Could you check a few things on this drawing? It's one solid part, dimensions in mm from its lowest x, y, z. A direction names the side the tool comes from. Coordinates: 2 decimals unless noted, no trailing zeros. Order: outer loops, then holes, each group sorted by start corner. A loop starts at its lowest first (then second) coordinate and runs counter-clockwise, first axis right, second up.
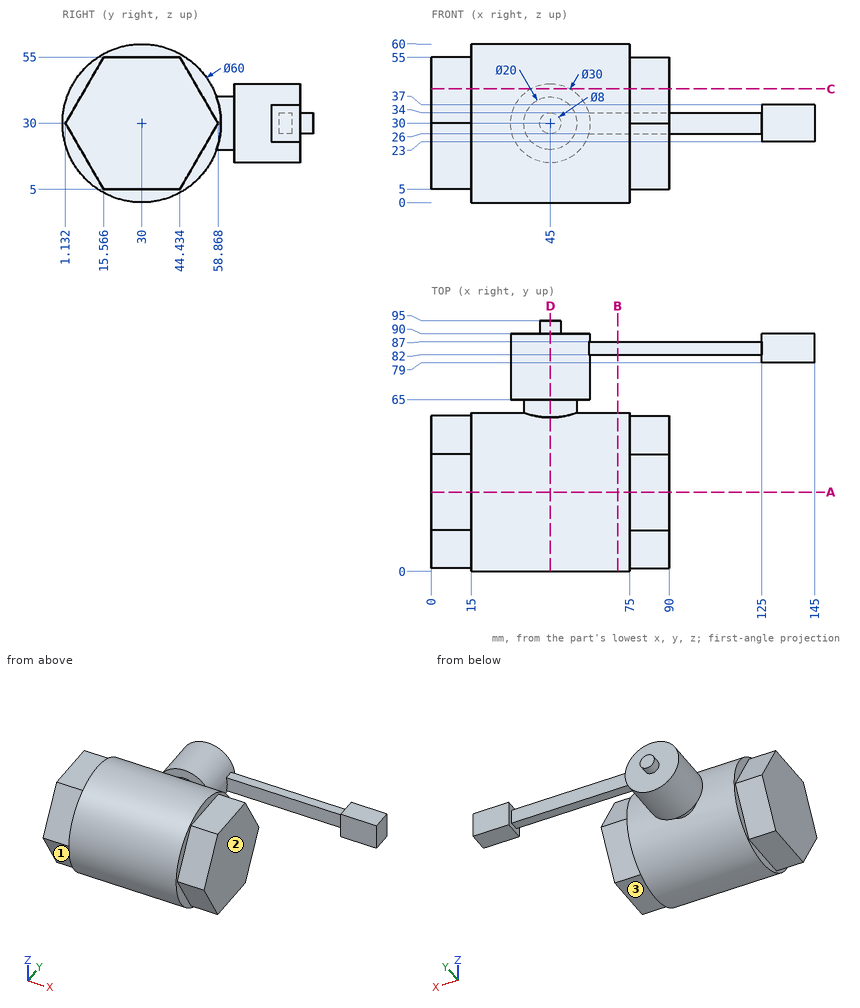
1. Imagine slicing it at C-C on z = 43. Please give me the cut outline in (x, y), then the cut area to 3 significant figures.
Completed:
outline: (0, 8.64) - (15, 8.64) - (15, 2.96) - (75, 2.96) - (75, 8.64) - (90, 8.64) - (90, 51.36) - (75, 51.36) - (75, 57.04) - (15, 57.04) - (15, 51.36) - (0, 51.36) - close; (37.52, 65) - (52.48, 65) - (52.48, 90) - (37.52, 90) - close
area: 4,900 mm2
2. Imagine slicing it at B-B on x = 70.5. Please give me the cut outline in (y, z).
Completed:
outline: circle Ø60 at (30, 30); (82, 26) - (87, 26) - (87, 34) - (82, 34) - close
3. Imagine slicing it at A-A on y = 30. Please give me the cut outline in (x, z).
Completed:
outline: (0, 5) - (15, 5) - (15, 0) - (75, 0) - (75, 5) - (90, 5) - (90, 55) - (75, 55) - (75, 60) - (15, 60) - (15, 55) - (0, 55) - close
4. Please list where these lines run through material, in increasing order: probe 1 along Z at (x, y) = (113, 86); probe 2 along Y at (x, z) = (129.5, 32); probe 3 along X at (y, z) = (44.5, 54).
Completed:
probe 1: z = 26 to 34
probe 2: y = 79 to 90
probe 3: x = 0 to 90
5. Imagine slicing it at D-D on x = 45. Please give me the cut outline in (y, z) (1 decimal), then the cut area to 3 significant figures.
Completed:
outline: (58.3, 20) - (65, 20) - (65, 15) - (90, 15) - (90, 26) - (95, 26) - (95, 34) - (90, 34) - (90, 45) - (65, 45) - (65, 40) - (58.3, 40) arc R30 ccw (long way) to start
area: 3,730 mm2
6. On a 3-axis mill with a long thin cutter (end or side, diameter ignored), from which of +Z, -Z, +X, -X, +Y, -Y can I reach the whole of each face in a straight line? I mean the marked faces 1, 2 and 3. Say none if no direction works.
Completed:
face 1: -Z, -X, -Y
face 2: +Z, -Z, +X, -Y
face 3: -Z, +X, +Y, -Y
7. I'm going to push flat-ended pins straight in: pin 1 (16.5 mm diameter, centred on x = 82, y = 24, fed in from -Z) (1 decimal); pin 2 (4 mm diameter, centred on x = 69, y = 17, fed in from -Z); pin 3 (3.5 mm diameter, centred on x = 133.5, y = 85.5, fed in from -Z); pin 4 (2 mm diameter, centred on x = 98, z = 24.5, fed in from +Y). Where does each tip first touch, or does it pass through?
Completed:
pin 1: stops at z = 0
pin 2: stops at z = 2.09
pin 3: stops at z = 23
pin 4: passes through
